Can you work these out from the model? Positions are in its coordinate system, mm. Face numbers are marked on the shaded views. Give positions to 0.01 mm unless a question says otherwise; leave off trailing zeros. Write each loop counter-clockwise with the first axis right and the second up, starting at its lowest first coordinate (ties: lowest second). Pieces come first, ordered by that corner, then holes.
from build123d import *

# Parameters (mm, degrees)
SKETCH1_W                        = 840
SKETCH1_H                        = 140
BOSS_EXTRUDE1_DEPTH              = 90
SKETCH2_W                        = 130
SKETCH2_H                        = 80
CUT_EXTRUDE1_DEPTH               = 848.702778101
FILLET2_R                        = 10
FILLET4_R                        = 10
M24X2_0_TAPPED_HOLE1_D           = 22
M24X2_0_TAPPED_HOLE1_CSINK_D     = 24.05
M24X2_0_TAPPED_HOLE1_CSINK_ANGLE = 90
CUT_EXTRUDE2_REACH               = 453.774
SKETCH7_W                        = 127
SKETCH7_H                        = 40
BOSS_EXTRUDE2_REACH              = 436.195
SKETCH8_R                        = 7.5


with BuildPart() as part:
    # Sketch1 → Boss-Extrude1 (new body)
    with BuildSketch(Plane(origin=(0, 0, 0), x_dir=(1, 0, 0), z_dir=(0, 1, 0))):
        Rectangle(SKETCH1_W, SKETCH1_H)
    extrude(amount=BOSS_EXTRUDE1_DEPTH)

    # Sketch2 → Cut-Extrude1 (cut, through all)
    with BuildSketch(Plane(origin=(420, 0, 0), x_dir=(0, 0, -1), z_dir=(1, 0, 0))):
        with Locations((0, 45)):
            Rectangle(SKETCH2_W, SKETCH2_H)
    extrude(amount=-CUT_EXTRUDE1_DEPTH, mode=Mode.SUBTRACT)

    # Fillet2
    fillet2_edges = [part.edges().sort_by_distance(p)[0] for p in [
        (0, 0, -70),
        (0, 90, -70),
    ]]
    fillet(fillet2_edges, radius=FILLET2_R)

    # Fillet4
    fillet4_edges = [part.edges().sort_by_distance(p)[0] for p in [
        (0, 90, 70),
        (0, 0, 70),
    ]]
    fillet(fillet4_edges, radius=FILLET4_R)

    # M24x2.0 Tapped Hole1 (through all)
    with Locations(Plane(origin=(0, 90, 0), x_dir=(1, 0, 0), z_dir=(0, 1, 0))):
        with Locations((-55, 0), (170, 0), (-280, 0), (380, 0)):
            CounterSinkHole(M24X2_0_TAPPED_HOLE1_D / 2, M24X2_0_TAPPED_HOLE1_CSINK_D / 2, counter_sink_angle=M24X2_0_TAPPED_HOLE1_CSINK_ANGLE)

    # Sketch7 → Cut-Extrude2 (cut, up to next)
    with BuildSketch(Plane.XY.offset(70), mode=Mode.PRIVATE) as cut_extrude2_sk1:
        with Locations((-373.5, 45)):
            Rectangle(SKETCH7_W, SKETCH7_H)
    cut_extrude2_tool1 = extrude(cut_extrude2_sk1.sketch, amount=-CUT_EXTRUDE2_REACH, mode=Mode.PRIVATE) & part.part
    add(cut_extrude2_tool1.solids().sort_by_distance((-373.5, 45, 70))[0], mode=Mode.SUBTRACT)

    # Sketch8 → Boss-Extrude2 (add, up to next)
    with BuildSketch(Plane(origin=(0, 5, 0), x_dir=(1, 0, 0), z_dir=(0, 1, 0)), mode=Mode.PRIVATE) as boss_extrude2_sk1:
        with Locations(Location((-370, -45, 0), (0, 0, 90))):
            Circle(SKETCH8_R)
    boss_extrude2_tool1 = extrude(boss_extrude2_sk1.sketch, amount=BOSS_EXTRUDE2_REACH, mode=Mode.PRIVATE) - part.part
    add(boss_extrude2_tool1.solids().sort_by_distance((-370, 5, 45))[0])


solid = part.part
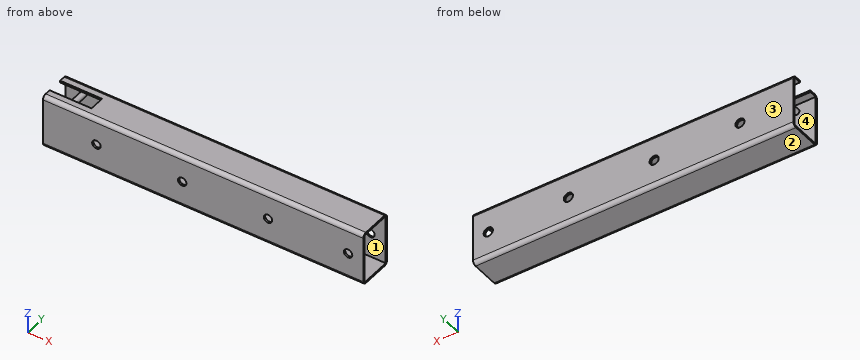
(1) Will these pins go through, and if not, where does the flat tip stop? P1, Ø4, axis at y = 52.5, z = 67, coming from the -X side; P2, Ø1.5, axis at x = -359.5, z = 68.5, coming from the +Y side; P3, Ø6, axis at x = 278.5, z = -4, coming from the -Y side; P4, Ø2.5, axis at x = -377, z = 67.5, coming from the -Y side.
Returned:
P1: stops at x = -310
P2: stops at y = 86.32
P3: stops at y = 0
P4: stops at y = 2.19
(2) Imagine slicing it at D-D, the plane x = -55. Write out the boundary of the cut face in (y, z) (3 decimals), plus the area to 3 significant figures.
Returned:
outline: (0, -60) arc R10 ccw to (10, -70) - (80, -70) arc R10 ccw to (90, -60) - (90, -12.025) - (88.975, -11) - (85, -11) - (85, -65) - (5, -65) - (5, -11) - (0, -11) - close; (0, 11) - (5, 11) - (5, 65) - (85, 65) - (85, 11) - (88.975, 11) - (90, 12.025) - (90, 60) arc R10 ccw to (80, 70) - (10, 70) arc R10 ccw to (0, 60) - close
area: 1,890 mm2
(3) Imagine slicing it at C-C, the plane z = -40. Write out the boundary of the cut face in (x, y), plus the area to 3 significant figures.
Returned:
outline: (-420, 0) - (420, 0) - (420, 5) - (-420, 5) - close; (-420, 85) - (420, 85) - (420, 90) - (-420, 90) - close
area: 8,400 mm2
(4) Imagine slicing it at A-A, the plane y = 17.5. Write out the boundary of the cut face in (x, z).
Returned:
outline: (-420, -70) - (420, -70) - (420, -65) - (-420, -65) - close; (-420, 65) - (420, 65) - (420, 70) - (-420, 70) - close; circle Ø15 at (-370, 45)
(5) If I drill on L1, parallel to Y at x = 229, z = -44.5; L2, parallel to Y at x = -359.5, z = 61.5; L3, parallel to Z at x = 295.5, y = 25, over which ranges is the centre line in solid material (lowest first)?
Returned:
L1: y = 0 to 5, 85 to 90
L2: y = 0.11 to 5, 85 to 89.89
L3: z = -70 to -65, 65 to 70
(6) Imagine slicing it at B-B, the plane x = -370. Write out the boundary of the cut face in (y, z), plus the area to 3 significant figures.
Returned:
outline: (0, -60) arc R10 ccw to (10, -70) - (80, -70) arc R10 ccw to (90, -60) - (90, 60) arc R10 ccw to (80, 70) - (65, 70) - (65, 65) - (85, 65) - (85, 52.5) - (5, 52.5) - (5, 65) - (25, 65) - (25, 70) - (10, 70) arc R10 ccw to (0, 60) - close; hole (5, -65) - (85, -65) - (85, 37.5) - (5, 37.5) - close
area: 3,110 mm2
(7) If we mould it in two halves opening along Z, with no side actions, what happens to the marked faces 1, 2, 3 and 4? For each: +Z half, -Z half, draft (parallel to the pull), parting line (faces both ways), or undercut.
Returned:
face 1: undercut
face 2: -Z half
face 3: draft
face 4: undercut
